```python
from build123d import *

# Parameters (mm, degrees)
F0_W          = 6.4
F0_H          = 6.5
F0_W_2        = 4
F0_H_2        = 2.5
F1_DEPTH      = 3.75
F2_SIZE2      = 5.3693575035
F2_SIZE       = 3.1
F3_W          = 10.5
F3_H          = 10.5
F4_DEPTH      = 1.5
F6_DEPTH      = 11
F6_DEPTH_BACK = 0.2
F7_R          = 0.5


with BuildPart() as f1:
    # F0 (on Right) → F1 (new body, symmetric)
    with BuildSketch(Plane.YZ):
        Polygon((15.24, 0), (15.24, 2.5), (8.84, 2.5), (-37.56, 2.5), (-37.56, 0), align=None)
        with Locations((12.04, 5.75)):
            Rectangle(F0_W, F0_H)
        with Locations((-39.56, 1.25)):
            Rectangle(F0_W_2, F0_H_2)
    extrude(amount=F1_DEPTH, both=True)

    # F2
    f2_edges = [f1.edges().sort_by_distance(p)[0] for p in [
        (-3.75, 8.84, 5.75),
    ]]
    f2_side = f1.faces().sort_by_distance((-3.75, -7.450196, 2.269608))[0]
    chamfer(f2_edges, length=F2_SIZE, length2=F2_SIZE2, reference=f2_side)

    # F3 (on face) → F4 (join)
    with BuildSketch(Plane(origin=(0, 15.24, 0), x_dir=(-1, 0, 0), z_dir=(0, 1, 0))):
        with Locations((0, 5.25)):
            Rectangle(F3_W, F3_H)
    extrude(amount=F4_DEPTH)

    # F5 (on Front) → F6 (cut, two sides)
    with BuildSketch(Plane.XZ) as f6_sk:
        with BuildLine():
            ThreePointArc((-0.8610377228, 2.0787289482), (-1.8708066277, 1.2500330243), (-2.25, 0))
            Line((-2.25, 0), (-0.8610377228, 0))
            Line((-0.8610377228, 0), (-0.8610377228, 2.0787289482))
        make_face()
        with BuildLine():
            Line((-0.8610377228, 4.6336889094), (-0.8610377228, 2.0787289482))
            ThreePointArc((-0.8610377228, 2.0787289482), (0, 2.25), (0.8610377228, 2.0787289482))
            Line((0.8610377228, 2.0787289482), (0.8610377228, 4.6336889094))
            Line((0.8610377228, 4.6336889094), (-0.8610377228, 4.6336889094))
        make_face()
        with BuildLine():
            ThreePointArc((0.8610377228, 2.0787289482), (0, 2.25), (-0.8610377228, 2.0787289482))
            Line((-0.8610377228, 2.0787289482), (-0.8610377228, 0))
            Line((-0.8610377228, 0), (0.8610377228, 0))
            Line((0.8610377228, 0), (0.8610377228, 2.0787289482))
        make_face()
        with BuildLine():
            ThreePointArc((2.25, 0), (1.8708066277, 1.2500330243), (0.8610377228, 2.0787289482))
            Line((0.8610377228, 2.0787289482), (0.8610377228, 0))
            Line((0.8610377228, 0), (2.25, 0))
        make_face()
    extrude(amount=F6_DEPTH, mode=Mode.SUBTRACT)
    extrude(f6_sk.sketch, amount=-F6_DEPTH_BACK, mode=Mode.SUBTRACT)

    # F7
    f7_edges = [f1.edges().sort_by_distance(p)[0] for p in [
        (-3.75, -13.16, 0),
        (-3.75, -14.81, 2.5),
        (3.75, -16.36, 2.5),
        (3.75, -13.16, 0),
    ]]
    fillet(f7_edges, radius=F7_R)


solid = f1.part
```
Here's how the part is built. I have some questions about the finished solid (model axes, mm). A direction names the side the tool comes from. Coordinates: 2 decimals unless noted, no trailing zeros. Write each loop counter-clockwise with the first axis right and the second up, starting at its lowest first coordinate (ties: lowest second). Pieces come first, ordered by that corner, then holes. Notation, with made-up numbers: (-19.5, 35) - (35.5, 35) arc R30 ccw to (35.5, 69) - close; hole circle Ø6 at (-36, 23). An arc over 180 degrees is marked (long way). One line per item, written item: value.
1) On a 3-axis mill with a long thin cutter (end or side, diameter ignored), from which of +Z, -Z, +X, -X, +Y, -Y can I reach the whole of each face in a straight line? I mean faces 4 (the flat face through (3.75, -5, 1)), 5 (the cylindrical face through (-1.86, -5.322, 1.265)), 6 (the flat face through (-3.75, -7, 1)). Say none if no direction works.
Model answer:
face 4: +Z, -Z, +X, -Y
face 5: -Z
face 6: +Z, -Z, -X, -Y
2) I need wall thicknesses on line 1 along Y through (x, z) = (4.5, 9.75); line 2 along Z through (x, y) = (0.25, -28); line 3 along Y through (x, z) = (-1, 1.5). Which ranges of each line are inside material? Lowest first, please.
Model answer:
line 1: y = 15.24 to 16.74
line 2: z = 0 to 2.5
line 3: y = -41.56 to -11, 0.2 to 16.74
3) Suppose I cut it at A-A on y = -9. Write out the boundary of the cut face in (x, z), and give its area (3 significant figures).
Model answer:
outline: (-3.75, 0.5) arc R0.5 ccw to (-3.25, 0) - (-2.25, 0) arc R2.25 cw to (-0.86, 2.08) - (-0.86, 2.5) - (-3.25, 2.5) arc R0.5 ccw to (-3.75, 2) - close; (0.86, 2.08) arc R2.25 cw to (2.25, 0) - (3.25, 0) arc R0.5 ccw to (3.75, 0.5) - (3.75, 2) arc R0.5 ccw to (3.25, 2.5) - (0.86, 2.5) - close
area: 10.1 mm²
4) Suppose I cut it at B-B on z = 7.75. Write out the boundary of the cut face in (x, y).
Model answer:
outline: (-5.25, 15.24) - (-3.75, 15.24) - (-3.75, 11.94) - (1.62, 8.84) - (3.75, 8.84) - (3.75, 15.24) - (5.25, 15.24) - (5.25, 16.74) - (-5.25, 16.74) - close
5) Suppose I cut it at D-D on z = 1.5. Write out the boundary of the cut face in (x, y), and give its area (3 significant figures).
Model answer:
outline: (-5.25, 15.24) - (-3.75, 15.24) - (-3.75, -41.56) - (3.75, -41.56) - (3.75, 15.24) - (5.25, 15.24) - (5.25, 16.74) - (-5.25, 16.74) - close; hole (-1.68, -11) - (1.68, -11) - (1.68, 0.2) - (-1.68, 0.2) - close
area: 404 mm²
6) Suppose I cut it at C-C on y = 3. Write out the boundary of the cut face in (x, z).
Model answer:
outline: (-3.75, 0.5) arc R0.5 ccw to (-3.25, 0) - (3.25, 0) arc R0.5 ccw to (3.75, 0.5) - (3.75, 2) arc R0.5 ccw to (3.25, 2.5) - (-3.25, 2.5) arc R0.5 ccw to (-3.75, 2) - close
7) I'm going to push flat-ended pins straight in: P1, Ø0.5, axis at y = -5.5, z = 2.5, coming from the -X side; P2, Ø1.1, axis at x = 2.5, z = 7, coming from the -Y side; P3, Ø4, axis at y = -23.5, z = 5.5, coming from the -X side; P4, Ø3, axis at x = 1, y = -22, coming from the +Z side. Where does each tip first touch, or does it pass through?
Model answer:
P1: stops at x = -3.68
P2: stops at y = 8.84
P3: passes through
P4: stops at z = 2.5
8) We'd pull the mould along X, two halves only. Please class faces 1 (the cylindrical face through (1.881, -5.322, 1.235)), 2 (the flat face through (0, 13, 9)), 3 (the flat face through (-1.03, 10.37, 5.45)): pulls with the +X half, pulls with the -X half, needs draft (parallel to the pull), parting line crosses it, or undercut.
Model answer:
face 1: undercut
face 2: needs draft
face 3: pulls with the -X half
